Source: CAD feature listing. Evaluate the final solid. Frame: model axes, mm. A direction names the side the tool comes from. Round coordinates to 2 decimals unless told otherwise and drop trailing zeros. Order: outer loops, then holes, each group sorted by start corner. A loop starts at its lowest first (then second) coordinate and runs counter-clockwise, first axis right, second up. Notation, with made-up numbers: M 85,-13.5 L 126,-13.5 A15 ccw 126,-7.5 Z; hole C 54.5,72 d5. An arc over 180 degrees is marked long. Use one line per item in the form item = value. Start each with the question number.
Q1. Material intervals for probe 1 along Z at (x, y) = (-23.5, 29.5) (3 decimals); probe 2 along Y at (x, z) = (-27.5, 2.5); probe 3 along Y at (x, z) = (-26, 17.5), sorted ascending.
Q2. Section B-B (y = 49). Return the cut outline in (x, z).
Q3. Reachability of faces 1 (the flat face through (-25, 127.5, 0)), 2 (the cylindrical face through (-25.07, 25.475, -15.466)), 3 (the cylindrical face through (-23.885, 15.916, -21.284)) from +Z, -Z, +X, -X, +Y, -Y: full face, straight path, thin tool, end or side. Return the list, or none.
Q4. Section D-D (x = -28). Give the number of separate pieces and of enclosed holes in the cut face, plus the area to 3 significant figures.
Q5. Contact query for flat-ended pins moving along their axis: pin 1 (2 mm diameter, centred on x = -25, z = -7.5, fed in from -Y); pin 2 (3 mm diameter, centred on x = -25, z = -22.5, fed in from +Y); pin 3 (18 mm diameter, centred on y = 100, z = 0, fed in from -X). Output: stop coordinate, or through.
Q6. Pull-direction query (Y, two-part tool) for faces 4 (the flat face through (-25, 61, -13.975)), 5 (the flat face through (-30, 68, 0)), 6 (the flat face through (-25, 10, 0)); classes: pulls with the +Y half, pulls with the -Y half, needs draft (parallel to the pull), parting line crosses it, or undercut.
Q7. Section C-C (z = -7.5). Return the cut outline in (x, y).
Q8. Section A-A (z = -22.5). Return the cut outline in (x, y).
from build123d import *

# Parameters (mm, degrees)
SKETCH_1_R          = 2
SKETCH_1_R_2        = 1.5
SKETCH_1_W          = 10
SKETCH_1_H          = 55
EXTRUDE_1_DEPTH     = 10
SKETCH_2_W          = 10
SKETCH_2_H          = 55
EXTRUDE_2_DEPTH     = 117.5
SKETCH_3_R          = 2.025
SKETCH_3_R_2        = 10
CUT_EXTRUDE_1_DEPTH = 143.543852901
CUT_EXTRUDE_2_DEPTH = 143.543852901
SKETCH_6_W          = 57.5
SKETCH_6_H          = 10
CUT_EXTRUDE_3_DEPTH = 143.060726452
SKETCH_7_R          = 1.65
CUT_EXTRUDE_4_DEPTH = 12


with BuildPart() as part:
    # 草图1 → 凸台-拉伸1 (new body)
    # profile 1 of 3: a face of its own
    with BuildSketch(Plane(origin=(0, 0, 0), x_dir=(1, 0, 0), z_dir=(0, 1, 0))):
        with BuildLine():
            ThreePointArc((0, -27.5), (27.5, 0), (0, 27.5))
            Line((0, 27.5), (-20, 27.5))
            Line((-20, 27.5), (-20, -27.5))
            Line((-20, -27.5), (0, -27.5))
        make_face()
        with Locations(Location((-15, -23.75, 0), (0, 0, 270))):
            Circle(SKETCH_1_R, mode=Mode.SUBTRACT)
        with Locations(Location((-8.876760389, -5.125, 0), (0, 0, 270))):
            Circle(SKETCH_1_R_2, mode=Mode.SUBTRACT)
        with Locations(Location((0, -10.25, 0), (0, 0, 270))):
            Circle(SKETCH_1_R_2, mode=Mode.SUBTRACT)
        with Locations(Location((8.876760389, -5.125, 0), (0, 0, 270))):
            Circle(SKETCH_1_R_2, mode=Mode.SUBTRACT)
        with Locations(Location((-8.876760389, 5.125, 0), (0, 0, 270))):
            Circle(SKETCH_1_R_2, mode=Mode.SUBTRACT)
        with Locations(Location((-15, 23.75, 0), (0, 0, 270))):
            Circle(SKETCH_1_R, mode=Mode.SUBTRACT)
        with Locations(Location((8.876760389, 5.125, 0), (0, 0, 270))):
            Circle(SKETCH_1_R_2, mode=Mode.SUBTRACT)
        with Locations(Location((0, 10.25, 0), (0, 0, 270))):
            Circle(SKETCH_1_R_2, mode=Mode.SUBTRACT)
    # profile 2 of 3: a face of its own
    with BuildSketch(Plane(origin=(0, 0, 0), x_dir=(1, 0, 0), z_dir=(0, 1, 0))):
        with BuildLine():
            ThreePointArc((0, -27.5), (27.5, 0), (0, 27.5))
            Line((0, 27.5), (-20, 27.5))
            Line((-20, 27.5), (-20, -27.5))
            Line((-20, -27.5), (0, -27.5))
        make_face()
        with Locations(Location((-15, -23.75, 0), (0, 0, 270))):
            Circle(SKETCH_1_R, mode=Mode.SUBTRACT)
        with Locations(Location((-8.876760389, -5.125, 0), (0, 0, 270))):
            Circle(SKETCH_1_R_2, mode=Mode.SUBTRACT)
        with Locations(Location((0, -10.25, 0), (0, 0, 270))):
            Circle(SKETCH_1_R_2, mode=Mode.SUBTRACT)
        with Locations(Location((8.876760389, -5.125, 0), (0, 0, 270))):
            Circle(SKETCH_1_R_2, mode=Mode.SUBTRACT)
        with Locations(Location((-8.876760389, 5.125, 0), (0, 0, 270))):
            Circle(SKETCH_1_R_2, mode=Mode.SUBTRACT)
        with Locations(Location((-15, 23.75, 0), (0, 0, 270))):
            Circle(SKETCH_1_R, mode=Mode.SUBTRACT)
        with Locations(Location((8.876760389, 5.125, 0), (0, 0, 270))):
            Circle(SKETCH_1_R_2, mode=Mode.SUBTRACT)
        with Locations(Location((0, 10.25, 0), (0, 0, 270))):
            Circle(SKETCH_1_R_2, mode=Mode.SUBTRACT)
    # profile 3 of 3: a face of its own
    with BuildSketch(Plane(origin=(0, 0, 0), x_dir=(1, 0, 0), z_dir=(0, 1, 0))):
        with Locations((-25, 0)):
            Rectangle(SKETCH_1_W, SKETCH_1_H)
    extrude(amount=EXTRUDE_1_DEPTH)

    # 草图2 → 凸台-拉伸2 (add)
    with BuildSketch(Plane(origin=(0, 10, 0), x_dir=(1, 0, 0), z_dir=(0, 1, 0))):
        with Locations((-25, 0)):
            Rectangle(SKETCH_2_W, SKETCH_2_H)
    extrude(amount=EXTRUDE_2_DEPTH)

    # 草图3 → 切除-拉伸1 (cut, through all)
    with BuildSketch(Plane.ZY.offset(30)):
        with Locations((-17.67766953, 117.67766953)):
            Circle(SKETCH_3_R)
        with Locations((17.67766953, 117.67766953)):
            Circle(SKETCH_3_R)
        with Locations((17.67766953, 82.32233047)):
            Circle(SKETCH_3_R)
        with Locations((-17.67766953, 82.32233047)):
            Circle(SKETCH_3_R)
        with Locations((0, 100)):
            Circle(SKETCH_3_R_2)
        with BuildLine():
            Line((-13.975, 63), (-13.975, 58))
            ThreePointArc((-13.975, 58), (-15.5, 56.475), (-17.025, 58))
            Line((-17.025, 58), (-17.025, 63))
            ThreePointArc((-17.025, 63), (-15.5, 64.525), (-13.975, 63))
        make_face()
        with BuildLine():
            Line((-13.975, 32), (-13.975, 27))
            ThreePointArc((-13.975, 27), (-15.5, 25.475), (-17.025, 27))
            Line((-17.025, 27), (-17.025, 32))
            ThreePointArc((-17.025, 32), (-15.5, 33.525), (-13.975, 32))
        make_face()
        with BuildLine():
            Line((13.975, 63), (13.975, 58))
            ThreePointArc((13.975, 58), (15.5, 56.475), (17.025, 58))
            Line((17.025, 58), (17.025, 63))
            ThreePointArc((17.025, 63), (15.5, 64.525), (13.975, 63))
        make_face()
        with BuildLine():
            Line((13.975, 32), (13.975, 27))
            ThreePointArc((13.975, 27), (15.5, 25.475), (17.025, 27))
            Line((17.025, 27), (17.025, 32))
            ThreePointArc((17.025, 32), (15.5, 33.525), (13.975, 32))
        make_face()
        with BuildLine():
            Line((11.05, 47.5), (11.05, 42.5))
            ThreePointArc((11.05, 42.5), (0, 31.45), (-11.05, 42.5))
            Line((-11.05, 42.5), (-11.05, 47.5))
            ThreePointArc((-11.05, 47.5), (0, 58.55), (11.05, 47.5))
        make_face()
    extrude(amount=-CUT_EXTRUDE_1_DEPTH, mode=Mode.SUBTRACT)

    # 草图5 → 切除-拉伸2 (cut, through all)
    with BuildSketch(Plane.ZY.offset(30)):
        Polygon((-27.5, 117.5), (-17.5, 127.5), (-27.5, 127.5), align=None)
        Polygon((27.5, 117.5), (27.5, 127.5), (17.5, 127.5), align=None)
    extrude(amount=-CUT_EXTRUDE_2_DEPTH, mode=Mode.SUBTRACT)

    # 草图6 → 切除-拉伸3 (cut, through all)
    with BuildSketch(Plane(origin=(0, 0, -27.5), x_dir=(-1, 0, 0), z_dir=(0, 0, -1))):
        with Locations((1.25, 5)):
            Rectangle(SKETCH_6_W, SKETCH_6_H)
    extrude(amount=-CUT_EXTRUDE_3_DEPTH, mode=Mode.SUBTRACT)

    # 草图7 → 切除-拉伸4 (cut)
    with BuildSketch(Plane.XZ.offset(-10)):
        with Locations(Location((-25, 22.5, 0), (0, 0, 270))):
            Circle(SKETCH_7_R)
        with Locations(Location((-25, 7.5, 0), (0, 0, 270))):
            Circle(SKETCH_7_R)
        with Locations(Location((-25, -7.5, 0), (0, 0, 270))):
            Circle(SKETCH_7_R)
        with Locations(Location((-25, -22.5, 0), (0, 0, 270))):
            Circle(SKETCH_7_R)
    extrude(amount=-CUT_EXTRUDE_4_DEPTH, mode=Mode.SUBTRACT)


solid = part.part
Results list:
q1.probe_1 = -27.5 to -17.025, -13.975 to 13.975, 17.025 to 27.5
q1.probe_2 = 10 to 31.74, 58.26 to 90.32, 109.68 to 127.5
q1.probe_3 = 10 to 80.31, 84.34 to 115.66, 119.69 to 127.5
q2.outline = M -30,-27.5 L -20,-27.5 L -20,-10.95 L -30,-10.95 Z; M -30,10.95 L -20,10.95 L -20,27.5 L -30,27.5 Z
q3.face_1 = +Z, -Z, +X, -X, +Y
q3.face_2 = +X, -X
q3.face_3 = -Y
q4.separate_pieces = 1
q4.enclosed_holes = 10
q4.area = 5,410 mm2
q5.pin_1 = 22
q5.pin_2 = 124
q5.pin_3 = through
q6.face_4 = undercut
q6.face_5 = needs draft
q6.face_6 = pulls with the -Y half
q7.outline = M -30,10 L -26.65,10 L -26.65,22 L -23.35,22 L -23.35,10 L -20,10 L -20,34.39 L -30,34.39 Z; M -30,55.61 L -20,55.61 L -20,93.39 L -30,93.39 Z; M -30,106.61 L -20,106.61 L -20,127.5 L -30,127.5 Z
q8.outline = M -30,10 L -26.65,10 L -26.65,22 L -23.35,22 L -23.35,10 L -20,10 L -20,122.5 L -30,122.5 Z
